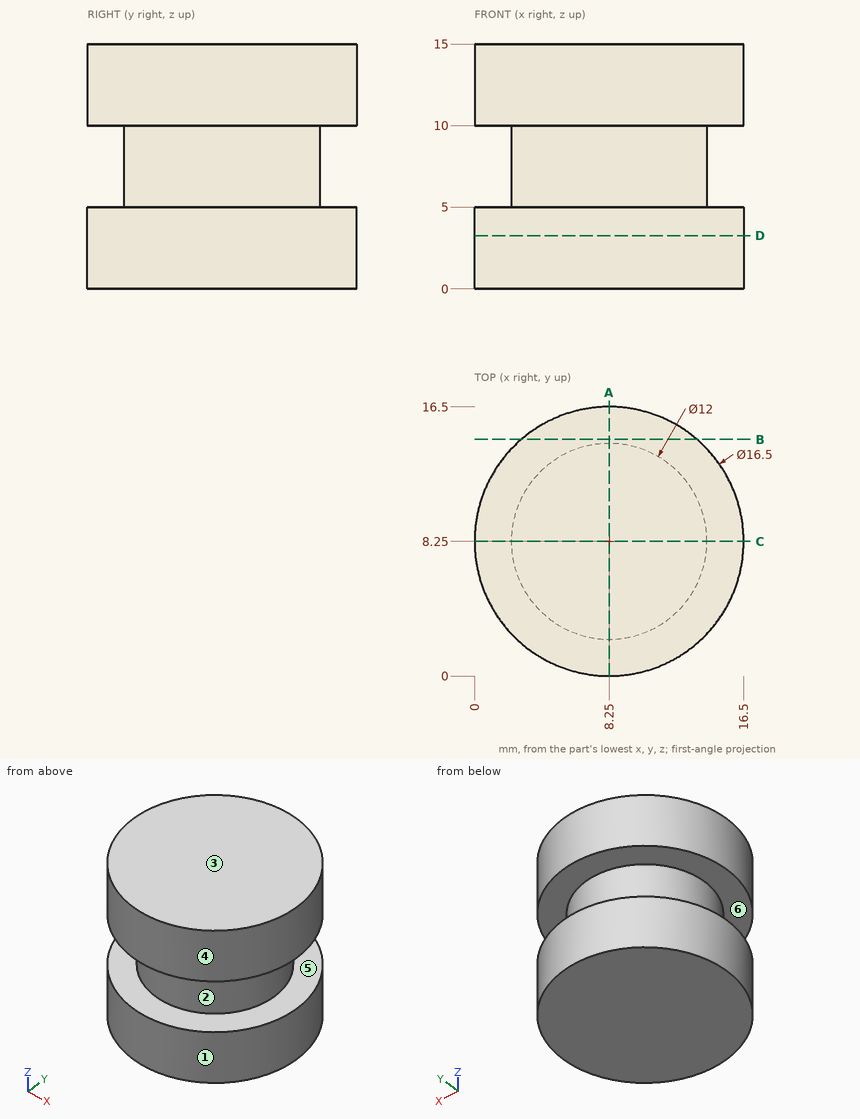
Geometry check sheet. Reference: drawing and pictorial views, mm from the part's lowest x, y, z. A direction names the side the tool comes from. Coordinates: 2 decimals unless noted, no trailing zeros. Loops run counter-clockwise (first coordinate to the right, second up) from the corner with the lowest first, then second, coordinate; pieces in that order, holes last.
1) Release check for a two-part mould opening along Z. For the marked faces 3, 4, 5 and 6 record: released by +Z, released by -Z, zero draft, split by the parting line, or undercut.
2) Sectioned sample at B-B (y = 14.5). Record the boundary of the cut face in (x, z).
3) Access from +Z, -Z, +X, -X, +Y, -Y to the whole of each face (thin tool, end or side, straight path). Record for the marked faces 1 and 2.
4) Gauge pin test, flat ends, axial feed: pin 1 (2 mm diameter, centred on y = 12.5, z = 13.5, fed in from +X); pin 2 (4 mm diameter, centred on x = 13, z = 9.5, fed in from +Y). Record the tip position at first contact, or that the pin passes through.
5) Sectioned sample at D-D (z = 3.25). Record the boundary of the cut face in (x, y), and give its area (3 significant figures).
6) Sectioned sample at A-A (x = 8.25). Record the boundary of the cut face in (y, z), and give its area (3 significant figures).
7) Material ranges on probe 1 along Z at (x, y) = (0.75, 8.5); probe 2 along Y at (x, z) = (2, 14.5); probe 3 along X at (y, z) = (4.25, 5.5), recorded low to high.
Check sheet entries:
1. face 3: released by +Z
1. face 4: zero draft
1. face 5: undercut
1. face 6: undercut
2. outline: (2.86, 0) - (13.64, 0) - (13.64, 5) - (2.86, 5) - close; (2.86, 10) - (13.64, 10) - (13.64, 15) - (2.86, 15) - close
3. face 1: +Z, -Z
3. face 2: none
4. pin 1: stops at x = 15.83
4. pin 2: stops at y = 16.01
5. outline: circle Ø16.5 at (8.25, 8.25)
5. area: 214 mm2
6. outline: (0, 0) - (16.5, 0) - (16.5, 5) - (14.25, 5) - (14.25, 10) - (16.5, 10) - (16.5, 15) - (0, 15) - (0, 10) - (2.25, 10) - (2.25, 5) - (0, 5) - close
6. area: 225 mm2
7. probe 1: z = 0 to 5, 10 to 15
7. probe 2: y = 2.86 to 13.64
7. probe 3: x = 3.78 to 12.72
